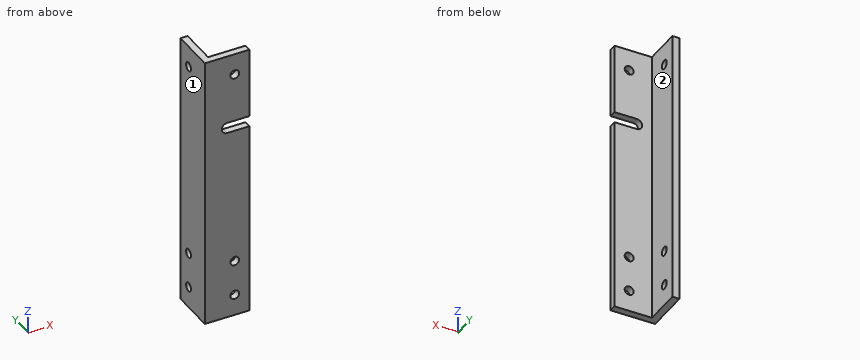
from build123d import *

# Parameters (mm, degrees)
EXTRUDE_1_DEPTH     = 155
HOLE_WIZARD_M6_1_D  = 5
HOLE_WIZARD_M6_2_D  = 5
CUT_EXTRUDE_1_DEPTH = 159.981130956


with BuildPart() as part:
    # 草图1 → 凸台-拉伸1 (new body)
    with BuildSketch(Plane.XY):
        Polygon((0, 25), (0, 0), (25, 0), (25, 4), (4, 4), (4, 25), align=None)
    extrude(amount=EXTRUDE_1_DEPTH)

    # M6 螺纹孔1 (through all)
    with Locations(Plane(origin=(0, 4, 0), x_dir=(1, 0, 0), z_dir=(0, 1, 0))):
        with Locations((16.75, -12), (16.75, -143), (16.75, -32)):
            Hole(HOLE_WIZARD_M6_1_D / 2)

    # M6 螺纹孔2 (through all)
    with Locations(Plane(origin=(4, 0, 0), x_dir=(0, 0, -1), z_dir=(1, 0, 0))):
        with Locations((-143, 16.75), (-12, 16.75), (-32, 16.75)):
            Hole(HOLE_WIZARD_M6_2_D / 2)

    # 草图6 → 切除-拉伸1 (cut, through all)
    with BuildSketch(Plane.XZ):
        with BuildLine():
            Line((25, 109.5), (12.5, 109.5))
            ThreePointArc((12.5, 109.5), (9.5, 112.5), (12.5, 115.5))
            Line((12.5, 115.5), (25, 115.5))
            ThreePointArc((25, 115.5), (28, 112.5), (25, 109.5))
        make_face()
    extrude(amount=-CUT_EXTRUDE_1_DEPTH, mode=Mode.SUBTRACT)


solid = part.part
Work out the finished part from the listing and answer in its coordinate system (mm). Face numbers are marked on the shaded views. A direction names the side the tool comes from. Coordinates: 2 decimals unless noted, no trailing zeros. Loops run counter-clockwise (first coordinate to the right, second up) from the corner with the lowest first, then second, coordinate; pieces in that order, holes last. Notation, with made-up numbers: (21.5, -16) -> (39.5, -16) arc R20 ccw to (39.5, -12) -> close; hole circle Ø2 at (20, 82). An arc over 180 degrees is marked (long way). Answer as CSV lines item,"result".
1) The part is cut by section D-D (x = 2.25). Give the vertices of the cut face in (y, z), and give its area (3 significant figures).
A:
outline,"(0, 0) -> (25, 0) -> (25, 155) -> (0, 155) -> close; hole circle Ø5 at (16.75, 12); hole circle Ø5 at (16.75, 32); hole circle Ø5 at (16.75, 143)"
area,"3,820 mm²"
2) The part is cut by section C-C (z = 143). Give the vertices of the cut face in (x, y).
A:
outline,"(0, 0) -> (14.25, 0) -> (14.25, 4) -> (4, 4) -> (4, 14.25) -> (0, 14.25) -> close; (0, 19.25) -> (4, 19.25) -> (4, 25) -> (0, 25) -> close; (19.25, 0) -> (25, 0) -> (25, 4) -> (19.25, 4) -> close"
3) The part is cut by section B-B (x = 16.75). Give the vertices of the cut face in (y, z).
A:
outline,"(0, 0) -> (4, 0) -> (4, 9.5) -> (0, 9.5) -> close; (0, 14.5) -> (4, 14.5) -> (4, 29.5) -> (0, 29.5) -> close; (0, 34.5) -> (4, 34.5) -> (4, 109.5) -> (0, 109.5) -> close; (0, 115.5) -> (4, 115.5) -> (4, 140.5) -> (0, 140.5) -> close; (0, 145.5) -> (4, 145.5) -> (4, 155) -> (0, 155) -> close"
4) Straight lines are drawn through the part: probe 1 along Z at (x, y) = (16.75, 3.25); probe 2 along X at (y, z) = (2.4, 143). For each, find the intervals that lie inside material, in ascending order.
A:
probe 1,"z = 0 to 9.5, 14.5 to 29.5, 34.5 to 109.5, 115.5 to 140.5, 145.5 to 155"
probe 2,"x = 0 to 14.25, 19.25 to 25"
5) The part is cut by section A-A (y = 2.5). Give the vertices of the cut face in (x, z).
A:
outline,"(0, 0) -> (25, 0) -> (25, 109.5) -> (12.5, 109.5) arc R3 cw to (12.5, 115.5) -> (25, 115.5) -> (25, 155) -> (0, 155) -> close; hole circle Ø5 at (16.75, 12); hole circle Ø5 at (16.75, 32); hole circle Ø5 at (16.75, 143)"
6) Flat-ended cylindrical pins translate along their axes: pin 1 (4.5 mm diameter, centred on x = 19, y = 2, fed in from -Z); pin 2 (6.5 mm diameter, centred on x = 16.75, z = 143, fed in from +Y); pin 3 (1 mm diameter, centred on y = 19.5, z = 80.5, fed in from +X). Find the tip coordinate at first contact, or state that the pin passes through.
A:
pin 1,"stops at z = 0"
pin 2,"stops at y = 4"
pin 3,"stops at x = 4"
7) For the marked faces 1 and 2, determine the directions among +Z, -Z, +X, -X, +Y, -Y from which every point of the face is accessible in a straight line to the end or side of a thin tool.
A:
face 1,"+Z, -Z, -X, +Y, -Y"
face 2,"+Z, -Z, +X, +Y"
